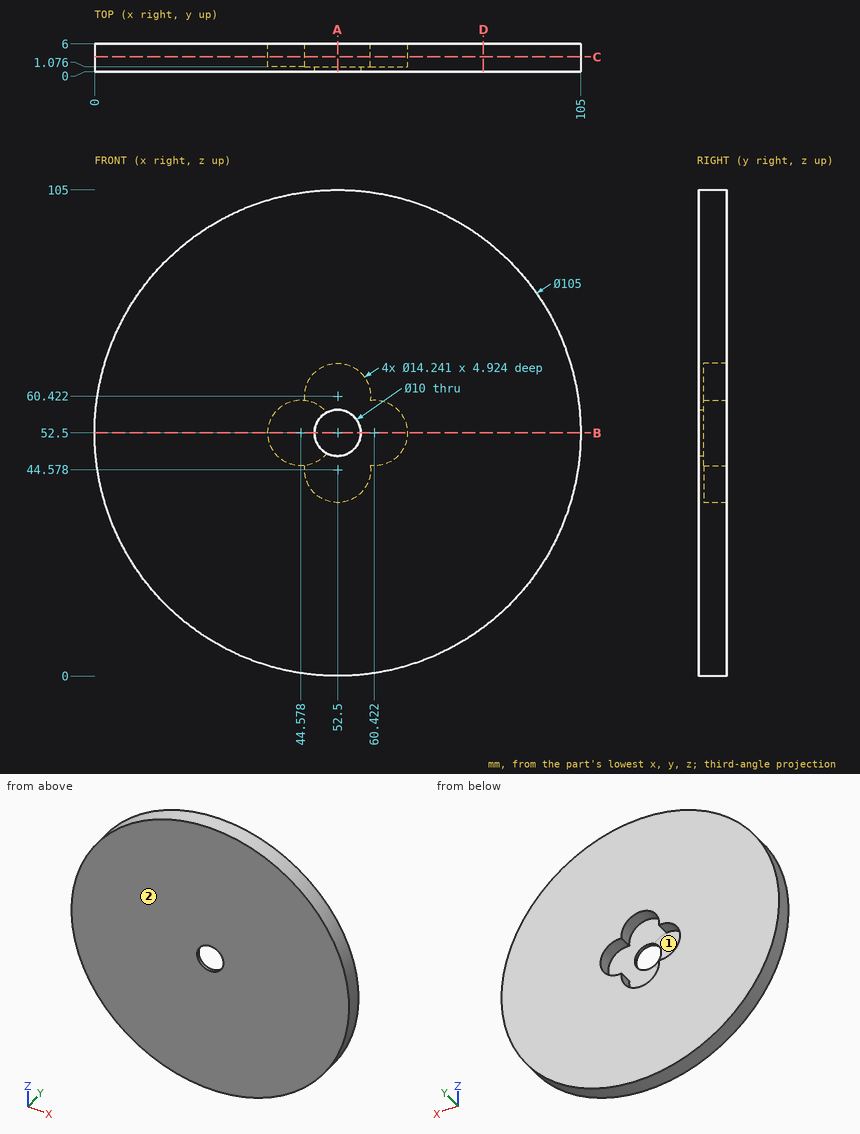
Could you check a few things on this drawing? It's one solid part, dimensions in mm from its lowest x, y, z. Round coordinates to 2 decimals unless told otherwise and drop trailing zeros. Loops run counter-clockwise (first coordinate to the right, second up) from the corner with the lowest first, then second, coordinate; pieces in that order, holes last. Notation, with made-up numbers: M 18.5,54.5 L 48.5,54.5 A29 cw 48.5,81.5 Z; hole C 35.25,13.25 d11. An arc over 180 degrees is marked long. Write each question's results on one line, items separated by ' | '. Start each with the question number.
(1) I want a section at D-D (x = 84). Please give me the cut outline in (y, z), then the cut area to 3 significant figures.
(2) Thinking about a two-plate mould opening in X: for the marked faces 1 and 2, which applies, pulls with the +X half, pulls with the -X half, needs draft (parallel to the pull), parting line crosses it, or undercut?
(3) If I drill on probe 1 along X at (y, z) = (2.6, 52.5); probe 2 along Z at (x, y) = (41, 1.6) (1 decimal), over which ranges is the centre line in solid material (lowest first)? Write a range as from..to.
(4) I want a section at B-B (z = 52.5). Please give me the cut outline in (x, y).
(5) I want a section at A-A (x = 52.5). Please give me the cut outline in (y, z).
(6) I want a section at C-C (y = 3.2). Please give me the cut outline in (x, z).
(7) Will these pins go through, and if not, where does the flat tip stop? P1, Ø3, axis at x = 92, y = 3.5, coming from the -Z side (1 decimal); P2, Ø1.5, axis at y = 4.5, z = 47, coming from the +X side (1 decimal); P3, Ø11.5, axis at x = 44.58, z = 52.5, coming from the +Y side.
Solved:
1) outline: M 0,10.5 L 6,10.5 L 6,94.5 L 0,94.5 Z | area: 504 mm²
2) face 1: undercut | face 2: needs draft
3) probe 1: x = 0..37.46, 67.54..105 | probe 2: z = 1.3..46.3, 58.7..103.7
4) outline: M 0,0 L 47.5,0 L 47.5,1.08 L 37.46,1.08 L 37.46,6 L 0,6 Z; M 57.5,0 L 105,0 L 105,6 L 67.54,6 L 67.54,1.08 L 57.5,1.08 Z
5) outline: M 0,0 L 6,0 L 6,37.46 L 1.08,37.46 L 1.08,47.5 L 0,47.5 Z; M 0,57.5 L 1.08,57.5 L 1.08,67.54 L 6,67.54 L 6,105 L 0,105 Z
6) outline: C 52.5,52.5 d105; hole M 45.43,45.43 A7.12 ccw long 59.57,45.43 A7.12 ccw long 59.57,59.57 A7.12 ccw long 45.43,59.57 A7.12 ccw long Z
7) P1: stops at z = 16.3 | P2: stops at x = 104.8 | P3: stops at y = 1.08
